Part model, mm, in its own coordinate system. Face numbers are marked on the shaded views. A direction names the side the tool comes from. Coordinates: 2 decimals unless noted, no trailing zeros. Loops run counter-clockwise (first coordinate to the right, second up) from the corner with the lowest first, then second, coordinate; pieces in that order, holes last. Notation, with made-up numbers: M -21.5,38 L 7.5,38 A27 ccw 7.5,66 Z; hole C -17.75,-36.75 d1. An arc over 180 degrees is marked long. Use a Markdown table: item, result. Add a question column.
1) Pin check, flat tip, straight feed: pin 1 Ø2 at (x, z) = (1, -1.5) entering from -Y. Stop position of the tip, or through.
2) Band-saw the part on A-A (x = 0.9). List the corners of the cut face in (y, z).
3) Band-saw the part on C-C (x = 2.55). List the corners of the cut face in (y, z), plus the area to 3 significant figures.
4) Band-saw the part on B-B (z = 12.5). List the corners of the cut face in (x, y).
5) Wall check: probe 1 along Y at (x, z) = (2.75, -2.25); probe 2 along X at (y, z) = (3.65, 11.75); probe 3 along Z at (x, y) = (0.25, 2.05). Give the ranges that are in metal, low to high. Write a range as from..to.
6) Pull direction Z, two halves, no side cores. Call the marked faces 3, 4 and 5: released by +Z, released by -Z, zero draft, split by the parting line, or undercut.
7) Band-saw the part on D-D (y = 1.4). List the corners of the cut face in (x, z), plus the area to 3 significant figures.
8) Tool access for the marked faces 1 and 2: list every direction of +Z, -Z, +X, -X, +Y, -Y with a clear straight run to the whole face (end or side of a thin tool).
Autodesk Inventor part; units mm, degrees
ref_plane "YZ Plane" through (0, 0, 0) normal (1, 0, 0) x (0, 1, 0)
ref_plane "XZ Plane" through (0, 0, 0) normal (0, 1, 0) x (-1, 0, 0)
ref_plane "XY Plane" through (0, 0, 0) normal (0, 0, 1) x (1, 0, 0)
sketch "Boceto1" plane through (0, 0, 0) normal (0, 1, 0) x (-1, 0, 0)
  line L0 (-3, -15) -> (3, -15)
  line L1 (3, -15) -> (3, 15)
  line L2 (3, 15) -> (-3, 15)
  line L3 (-3, 15) -> (-3, -15)
  line L4 (-3, -15) -> (3, 15) construction
  line L5 (3, -15) -> (-3, 15) construction
  circle A0 centre (0, 12.5) radius 1.5
  point P0 (0, 0)
  point P1 (0, 15)
  dimension "d0" = 6
  dimension "d1" = 30
  dimension "d3" = 3
  dimension "d12" = 2.5
extrude "Extrusión1" add sketch "Boceto1" along normal blind 5
chamfer "Chaflán1" distance 11 distance2 5 1 edges at (0, 5, -15) measured on face at (-0.0603, 5, -6.3297)
sketch "Boceto2" plane through (0, 0, 0) normal (0, -1, 0) x (1, 0, 0)
  line L0 (3, 15) -> (3, -15)
  line L1 (-3, -15) -> (-3, 15)
  line L2 (3, -15) -> (-3, -15)
  line L3 (-3, -15) -> (-3, -13)
  line L4 (-3, -13) -> (3, -13)
  line L5 (3, -13) -> (3, -15)
  point P0 (0, 0)
  point P1 (-3, -15)
  point P2 (3, -13)
  dimension "d9" = 2
extrude "Extrusión2" add sketch "Boceto2" along normal blind 1
properties part number "Soporte PCB pieza plastico"
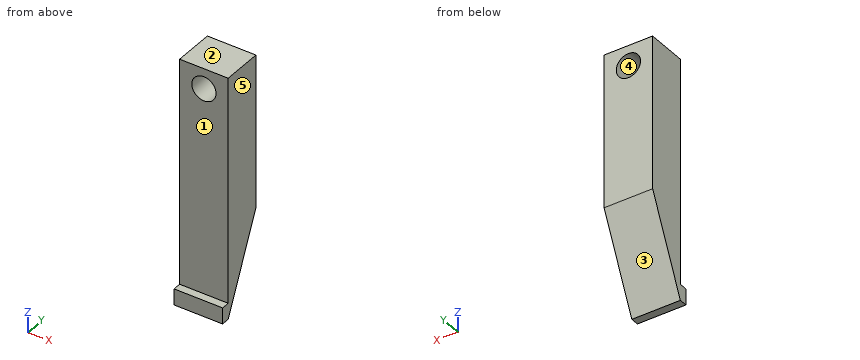
Entries:
| question | item | result |
|---|---|---|
| 1 | pin 1 | y = 0 |
| 2 | outline | M -1,-15 L 0,-15 L 5,-4 L 5,11.3 L 0,11.3 L 0,-13 L -1,-13 Z; M 0,13.7 L 5,13.7 L 5,15 L 0,15 Z |
| 3 | outline | M -1,-15 L 0,-15 L 5,-4 L 5,15 L 0,15 L 0,-13 L -1,-13 Z |
| 3 | area | 125 mm2 |
| 4 | outline | M -3,0 L -1.5,0 L -1.5,5 L -3,5 Z; M 1.5,0 L 3,0 L 3,5 L 1.5,5 Z |
| 5 | probe 1 | 0..5 |
| 5 | probe 2 | -3..-1.3, 1.3..3 |
| 5 | probe 3 | -10.49..11.02, 13.98..15 |
| 6 | face 3 | released by -Z |
| 6 | face 4 | undercut |
| 6 | face 5 | zero draft |
| 7 | outline | M -3,-11.92 L 3,-11.92 L 3,15 L -3,15 Z; hole C 0,12.5 d3 |
| 7 | area | 154 mm2 |
| 8 | face 1 | +Z, +X, -X, -Y |
| 8 | face 2 | +Z, +X, -X, +Y, -Y |
